Print and shaded views of the part. All mm, measured from the part's lowest x, y and z. Round coordinates to 2 decimals unless told otherwise and drop trailing zeros. Write each loop counter-clockwise with the first axis right and the second up, starting at its lowest first coordinate (ties: lowest second). Pieces come first, ordered by that corner, then holes. Notation, with made-up numbers: (-6.5, -8) - (28.5, -8) arc R21 cw to (28.5, 22) - close; hole circle Ø1 at (-32.75, 62.5). An arc over 180 degrees is marked (long way). Answer as a JSON object with one key per item and string values. Group by question number.
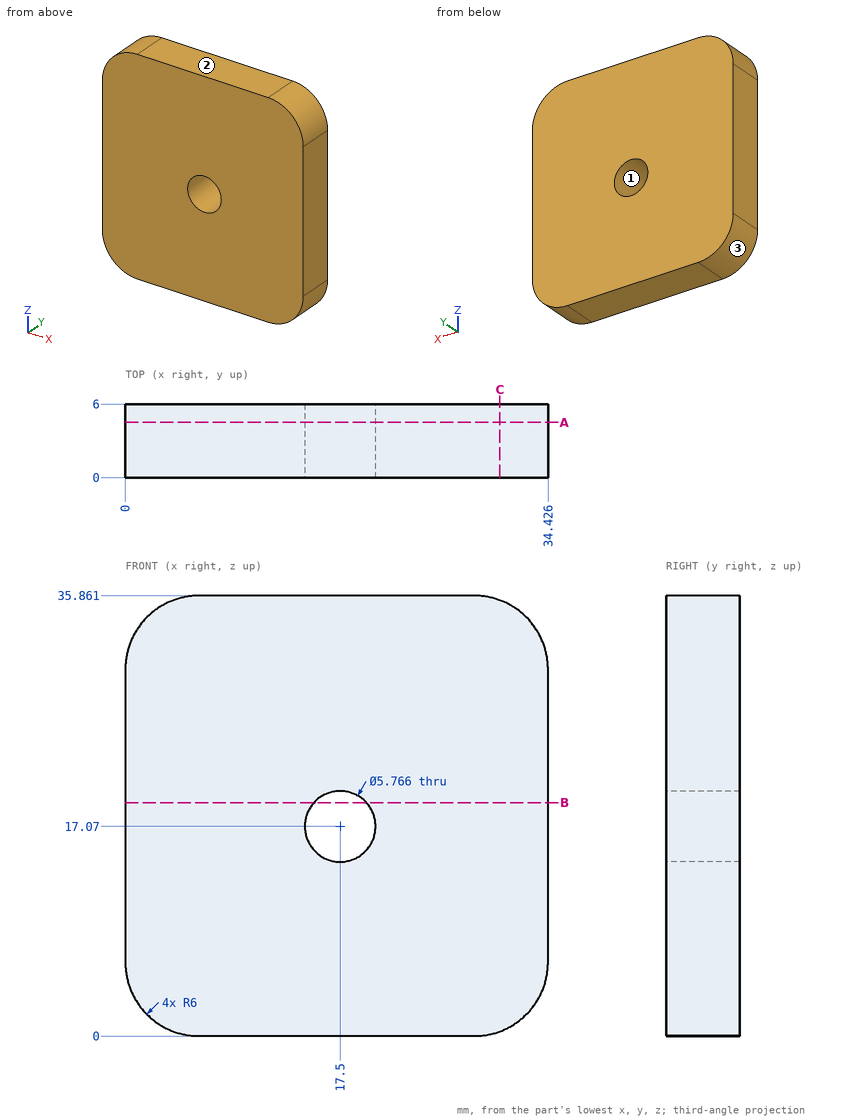
(1) Drill centre lines: line 1 (X direction, y = 0.7, z = 17.5); line 2 (Z direction, x = 18.5, y = 1.75) (1 decimal); line 3 (Z direction, x = 16, y = 4.9). Where is each one in solid material? Low to high. Write a range as from..to.
(2) Slice it at B-B (z = 19). Write the cut outline in (x, y).
(3) Pull direction Z, two halves, no side cores. Call the marked faces 1, 2 and 3: pulls with the +Z half, pulls with the -Z half, needs draft (parallel to the pull), parting line crosses it, or undercut.
(4) Slice it at C-C (x = 30.5). Write the cut outline in (y, z), then the cut area to 3 significant figures.
(5) Slice it at A-A (y = 4.5). Write the cut outline in (x, z).
Answer:
{
 "1": {"line 1": "0..14.65, 20.35..34.43", "line 2": "0..14.4, 19.8..35.9", "line 3": "0..14.61, 19.53..35.86"},
 "2": {"outline": "(0, 0) - (15.36, 0) - (15.36, 6) - (0, 6) - close; (19.64, 0) - (34.43, 0) - (34.43, 6) - (19.64, 6) - close"},
 "3": {"face 1": "undercut", "face 2": "pulls with the +Z half", "face 3": "pulls with the -Z half"},
 "4": {"outline": "(0, 0.37) - (6, 0.37) - (6, 35.49) - (0, 35.49) - close", "area": "211 mm²"},
 "5": {"outline": "(0, 6) arc R6 ccw to (6, 0) - (28.43, 0) arc R6 ccw to (34.43, 6) - (34.43, 29.86) arc R6 ccw to (28.43, 35.86) - (6, 35.86) arc R6 ccw to (0, 29.86) - close; hole circle Ø5.77 at (17.5, 17.07)"}
}
